Here's how the part is built. I have some questions about the finished solid (model axes, mm). A direction names the side the tool comes from. Give positions to 0.01 mm unless a question says otherwise; leave off trailing zeros. Order: outer loops, then holes, each group sorted by start corner. A loop starts at its lowest first (then second) coordinate and runs counter-clockwise, first axis right, second up. Notation, with made-up numbers: M 17.25,17.5 L 30.25,17.5 A10 cw 30.25,26.5 Z; hole C 20.25,62.5 d4. An arc over 180 degrees is marked long. Use one line per item in the form item = value.
from build123d import *

# Parameters (mm, degrees)
SKETCH_R     = 1.5
PAD_DEPTH    = 1.5
SKETCH001_R  = 1.5
PAD001_DEPTH = 3
SKETCH002_W  = 2
SKETCH002_H  = 15
PAD002_DEPTH = 11
SKETCH003_W  = 15.132667
SKETCH003_H  = 2
PAD003_DEPTH = 17
SKETCH004_W  = 15
SKETCH004_H  = 2
PAD004_DEPTH = 11
SKETCH005_W  = 15
SKETCH005_H  = 2
PAD005_DEPTH = 17


with BuildPart() as part:
    # Sketch → Pad (new body, symmetric)
    with BuildSketch(Plane.XZ):
        Polygon((28, -24), (28, -80), (-13, -80), (-13, 0), (9, 0), align=None)
        with Locations((18, -54)):
            Circle(SKETCH_R, mode=Mode.SUBTRACT)
        with Locations((2, -70)):
            Circle(SKETCH_R, mode=Mode.SUBTRACT)
    extrude(amount=PAD_DEPTH, both=True)

    # Sketch001 (on Face4 of Pad) → Pad001 (join)
    with BuildSketch(Plane(origin=(0, 0, 0), x_dir=(-1, 0, 0), z_dir=(0, 0, 1))):
        Polygon((-9, -1.5), (-3, -9.5), (13, -9.5), (13, -1.5), (6, 1.5), (6, 11.5), (-9, 11.5), (-9, 1.5), align=None)
        with Locations((0, -4.5)):
            Circle(SKETCH001_R, mode=Mode.SUBTRACT)
        with Locations((2, 7.33216)):
            Circle(SKETCH001_R, mode=Mode.SUBTRACT)
    extrude(amount=-PAD001_DEPTH)

    # Sketch002 (on Face5 of Pad001) → Pad002 (join)
    with BuildSketch(Plane.XZ.offset(1.5)):
        with Locations((27, -72.5)):
            Rectangle(SKETCH002_W, SKETCH002_H)
        with Locations((10, -72.5)):
            Rectangle(SKETCH002_W, SKETCH002_H)
    extrude(amount=PAD002_DEPTH)

    # Sketch003 (on Face21 of Pad002) → Pad003 (join)
    with BuildSketch(Plane(origin=(11, 0, 0), x_dir=(0, 0, 1), z_dir=(1, 0, 0))):
        with Locations((-72.433667, 11.5)):
            Rectangle(SKETCH003_W, SKETCH003_H)
    extrude(amount=PAD003_DEPTH)

    # Sketch004 (on Face4 of Pad003) → Pad004 (join)
    with BuildSketch(Plane(origin=(0, 1.5, 0), x_dir=(1, 0, 0), z_dir=(0, 1, 0))):
        with Locations((20.5, 79)):
            Rectangle(SKETCH004_W, SKETCH004_H)
        with Locations((20.5, 62)):
            Rectangle(SKETCH004_W, SKETCH004_H)
    extrude(amount=PAD004_DEPTH)

    # Sketch005 (on Face17 of Pad004) → Pad005 (join)
    with BuildSketch(Plane(origin=(0, 0, -78), x_dir=(-1, 0, 0), z_dir=(0, 0, 1))):
        with Locations((-20.5, -11.5)):
            Rectangle(SKETCH005_W, SKETCH005_H)
    extrude(amount=PAD005_DEPTH)


solid = part.part
Q1. I want a section at A-A on z = -70. Write out the boundary of the cut face in (x, y), then the cut area to 3 significant figures.
Found:
outline = M -13,-1.5 L 0.5,-1.5 L 0.5,1.5 L -13,1.5 Z; M 3.5,-1.5 L 9,-1.5 L 9,-12.5 L 28,-12.5 L 28,1.5 L 3.5,1.5 Z; M 13,10.5 L 28,10.5 L 28,12.5 L 13,12.5 Z; hole M 11,-10.5 L 26,-10.5 L 26,-1.5 L 11,-1.5 Z
area = 218 mm²
Q2. Thinking about a two-plate mould opening in Z: for faces 4 (the face through (10, -7, -65)), 5 (the face through (0, 3, -1)), 6 (the face through (20, 6, -63)), 7 (the face through (19, -11, -80)), which applies, +Z half, -Z half, draft (parallel to the pull), parting line (faces both ways), or undercut?
Found:
face_4 = +Z half
face_5 = draft
face_6 = undercut
face_7 = -Z half
Q3. I'm going to push flat-ended pins straight in: pin 1 Ø4.5 at (y, z) = (-5.5, -70.5) entering from -X; pin 2 Ø8 at (x, z) = (-5, -19) entering from +Y; pin 3 Ø2.5 at (x, y) = (20, 4.5) entering from +Z. Where does each tip first touch, or does it pass through?
Found:
pin_1 = 9
pin_2 = 1.5
pin_3 = -61
Q4. I need wall thicknesses on L1, parallel to Y at x = 20, z = -70.5; L2, parallel to Y at x = -2, z = -1.4; L3, parallel to X at y = -4.5, z = -72. Which ranges of each line are inside material? Lowest first, please.
Found:
L1 = -12.5 to -10.5, -1.5 to 1.5, 10.5 to 12.5
L2 = -11.5 to -8.83, -5.83 to 9.5
L3 = 9 to 11, 26 to 28
Q5. On a 3-axis mill with a long thin cutter (end or side, diameter ignored), from which of +Z, -Z, +X, -X, +Y, -Y can I reach the whole of each face in a straight line? I mean faces 1 (the face through (13, 11, -71)), 2 (the face through (9, -7, -1)), 3 (the face through (26, -6, -73)). Say none if no direction works.
Found:
face_1 = +Z, -Z, -X, +Y
face_2 = +Z, +X, -Y
face_3 = +Z, -Z
Q6. I want a section at B-B on x = 18. Write out the boundary of the cut face in (y, z), then the cut area to 3 significant figures.
Found:
outline = M -12.5,-80 L -10.5,-80 L -10.5,-64.87 L -12.5,-64.87 Z; M -1.5,-80 L 12.5,-80 L 12.5,-61 L 1.5,-61 L 1.5,-55.5 L -1.5,-55.5 Z; M -1.5,-52.5 L 1.5,-52.5 L 1.5,-11.37 L -1.5,-11.37 Z; hole M 1.5,-78 L 10.5,-78 L 10.5,-63 L 1.5,-63 Z
area = 301 mm²
Q7. I want a section at D-D on z = -54. Write out the boundary of the cut face in (x, y), then the cut area to 3 significant figures.
Found:
outline = M -13,-1.5 L 16.5,-1.5 L 16.5,1.5 L -13,1.5 Z; M 19.5,-1.5 L 28,-1.5 L 28,1.5 L 19.5,1.5 Z
area = 114 mm²
Q8. I want a section at C-C on y = 4.5. Write out the boundary of the cut face in (x, z).
Found:
outline = M -13,-3 L -1.5,-3 L -1.5,0 L -13,0 Z; M 1.5,-3 L 6.75,-3 L 6.75,0 L 1.5,0 Z; M 13,-80 L 28,-80 L 28,-78 L 13,-78 Z; M 13,-63 L 28,-63 L 28,-61 L 13,-61 Z
